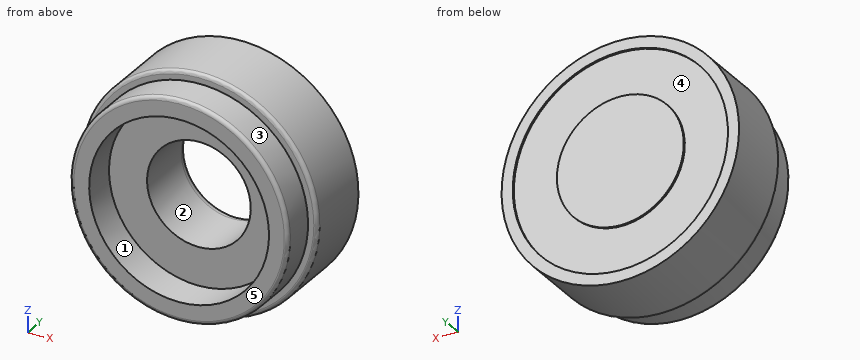
```python
from build123d import *

# Parameters (mm, degrees)
FILLET_1_R          = 1
SKETCH_4_R          = 28
SKETCH_4_R_2        = 16.5
CUT_EXTRUDE_1_DEPTH = 0.5
FILLET_2_R          = 3


with BuildPart() as part:
    # Эскиз3 → Повернуть2 (revolve)
    with BuildSketch(Plane.XY, mode=Mode.PRIVATE) as revolve_2_sk:
        Polygon((23.4, 0), (28.4, 0), (28.4, 9), (30.9, 9), (30.9, 27.5), (13.5, 27.5), (13.5, 9), (23.4, 9), align=None)
    revolve(revolve_2_sk.sketch.rotate(Axis((0, 0, 0), (0, 1, 0)), 90), axis=Axis((0, 0, 0), (0, 1, 0)))

    # Скругление1
    fillet_1_edges = [part.edges().sort_by_distance(p)[0] for p in [
        (0, 9, 30.9),
        (0, 0, 28.4),
    ]]
    fillet(fillet_1_edges, radius=FILLET_1_R)

    # Эскиз4 → Вырез-Вытянуть1 (cut)
    with BuildSketch(Plane(origin=(0, 27.5, 0), x_dir=(1, 0, 0), z_dir=(0, 1, 0))):
        with Locations(Location((0, 0, 0), (0, 0, 270))):
            Circle(SKETCH_4_R)
        with Locations(Location((0, 0, 0), (0, 0, 270))):
            Circle(SKETCH_4_R_2, mode=Mode.SUBTRACT)
    extrude(amount=-CUT_EXTRUDE_1_DEPTH, mode=Mode.SUBTRACT)

    # Скругление2
    fillet_2_edges = [part.edges().sort_by_distance(p)[0] for p in [
        (0, 27.5, 13.5),
    ]]
    fillet(fillet_2_edges, radius=FILLET_2_R - 0.0001)  # a hair under: the kernel refuses the full size


solid = part.part
```
Source: CAD feature listing. Evaluate the final solid. Frame: model axes, mm. Face numbers are marked on the shaded views. A direction names the side the tool comes from. Round coordinates to 2 decimals unless told otherwise and drop trailing zeros. Loops run counter-clockwise (first coordinate to the right, second up) from the corner with the lowest first, then second, coordinate; pieces in that order, holes last.
(1) Contact query for flat-ended pins moving along their axis: pin 1 Ø8 at (x, z) = (-2, 13) entering from +Y; pin 2 Ø10 at (x, y) = (24.5, 12.5) entering from +Z; pin 3 Ø10 at (x, y) = (6.5, 4.5) entering from -Z; pin 4 Ø3 at (x, y) = (5.5, 12) entering from -Z. Output: stop coordinate, or through.
From the geometry:
pin 1: stops at y = 27.5
pin 2: stops at z = 23.97
pin 3: stops at z = -30.2
pin 4: stops at z = -30.64
(2) Material intervals for probe 1 along Y at (x, z) = (19, -4); probe 2 along X at (y, z) = (14.5, 0); probe 3 along X at (y, z) = (2.25, 4.5), sorted ascending.
From the geometry:
probe 1: y = 9 to 27
probe 2: x = -30.9 to -13.5, 13.5 to 30.9
probe 3: x = -28.04 to -22.96, 22.96 to 28.04
(3) Section query C-C (y = 21.75). Output: boundary loops of the cut face in (x, z).
From the geometry:
outline: circle Ø61.8 at (0, 0); hole circle Ø27 at (0, 0)
(4) Access query for the marked faces 1 and 2. Directions: +Z, -Z, +X, -X, +Y, -Y. A direction counts if a zero-diameter tool reaches every point of the face in a straight line with its end or side. Return the directions, or none.
From the geometry:
face 1: -Y
face 2: +Y, -Y
(5) Pull-direction query (X, two-part tool) for the marked faces 3, 4 and 5; classes: +X half, -X half, draft (parallel to the pull), parting line (faces both ways), or undercut.
From the geometry:
face 3: parting line
face 4: undercut
face 5: draft
